The listing builds one solid part. Answer for the finished solid, in the listing's coordinates (mm). Give positions to 0.01 mm unless a question says otherwise; leave off trailing zeros. Write each loop counter-clockwise with the first axis right and the second up, starting at its lowest first coordinate (ties: lowest second). Pieces come first, ordered by that corner, then holes. Notation, with made-up numbers: M 4,81.5 L 43,81.5 A20 cw 43,106.5 Z; hole C 47,-24.5 d5. An arc over 180 degrees is marked long. Return JSON: item names as keys, results as strings.
from build123d import *

# Parameters (mm, degrees)
SKETCH1_R           = 2.5
BOSS_EXTRUDE1_DEPTH = 3
CUT_EXTRUDE1_DEPTH  = 4


with BuildPart() as part:
    # Sketch1 → Boss-Extrude1 (new body)
    with BuildSketch(Plane.XY):
        with BuildLine():
            Line((0.605, 10.983349899), (100.3025, 5.491674949))
            ThreePointArc((100.3025, 5.491674949), (105.5, 0), (100.3025, -5.491674949))
            Line((100.3025, -5.491674949), (0.605, -10.983349899))
            ThreePointArc((0.605, -10.983349899), (-11, 0), (0.605, 10.983349899))
        make_face()
        with Locations((100, 0)):
            Circle(SKETCH1_R, mode=Mode.SUBTRACT)
    extrude(amount=BOSS_EXTRUDE1_DEPTH)

    # Sketch2 → Cut-Extrude1 (cut, through all)
    with BuildSketch(Plane.XY.offset(3)):
        with BuildLine():
            Line((1.9, 1.46628783), (1.9, -1.46628783))
            ThreePointArc((1.9, -1.46628783), (-2.4, 0), (1.9, 1.46628783))
        make_face()
    extrude(amount=-CUT_EXTRUDE1_DEPTH, mode=Mode.SUBTRACT)


solid = part.part
Item 1: A cutting plane is placed at B-B, the plane z = 0.65. Write down the section's boundary in (x, y) (1 decimal).
Geometry results:
{"outline": "M 0.6,-11 L 100.3,-5.5 A5.5 ccw 100.3,5.5 L 0.6,11 A11 ccw long Z; hole M 1.9,-1.5 L 1.9,1.5 A2.4 ccw long Z; hole C 100,0 d5"}
Item 2: Find the intervals of material crossed by line 1 (X direction, y = -0.5, z = 0.8); line 2 (Y direction, x = 0, z = 1.15); line 3 (X direction, y = -1, z = 0.65), in increasing order.
Geometry results:
{"line 1": "x = -10.99 to -2.35, 1.9 to 97.55, 102.45 to 105.48", "line 2": "y = -11 to -2.4, 2.4 to 11", "line 3": "x = -10.95 to -2.18, 1.9 to 97.71, 102.29 to 105.41"}
Item 3: A cutting plane is placed at C-C, the plane x = 44.5. Write down the section's boundary in (y, z).
Geometry results:
{"outline": "M -8.57,0 L 8.57,0 L 8.57,3 L -8.57,3 Z"}
Item 4: Determine the mould class of faces 1 (the cylindrical face through (-11, 0, 1)), 2 (the cylindrical face through (102.385, 0.751, 1.479)), 3 (the flat face through (1.9, 0, 2)), 4 (the flat face through (35, 0, 0)) for opening direction Y: +Y half, -Y half, draft (parallel to the pull), parting line (faces both ways), or undercut.
Geometry results:
{"face 1": "parting line", "face 2": "undercut", "face 3": "undercut", "face 4": "draft"}
Item 5: A cutting plane is placed at D-D, the plane y = -6.5. Write down the section's boundary in (x, z).
Geometry results:
{"outline": "M -8.87,0 L 82,0 L 82,3 L -8.87,3 Z"}
Item 6: A cutting plane is placed at A-A, the plane y = 0. Write down the section's boundary in (x, z), plus the area to 3 significant figures.
Geometry results:
{"outline": "M -11,0 L -2.4,0 L -2.4,3 L -11,3 Z; M 1.9,0 L 97.5,0 L 97.5,3 L 1.9,3 Z; M 102.5,0 L 105.5,0 L 105.5,3 L 102.5,3 Z", "area": "322 mm2"}
